Part model, mm, in its own coordinate system. A direction names the side the tool comes from. Round coordinates to 2 decimals unless told otherwise and drop trailing zeros. Write each loop counter-clockwise with the first axis right and the second up, starting at its lowest first coordinate (ties: lowest second). Pieces come first, ordered by that corner, then holes. Notation, with made-up numbers: M 88.25,63 L 128.25,63 A20 cw 128.25,79 Z; hole C 19,-16 d10. An arc over 180 degrees is marked long. Answer as a JSON object with one key per item and string values. Group by question number.
1. Band-saw the part on B-B, the plane x = 84. Write the cut outline in (y, z), plus the area to 3 significant figures.
2. Band-saw the part on A-A, the plane z = 8.25. Write the cut outline in (x, y).
3. Band-saw the part on C-C, the plane y = 62.5. Write the cut outline in (x, z), plus the area to 3 significant figures.
4. Drill centre lines: line 1 (Y direction, x = 192.5, z = 6.25); line 2 (X direction, y = 66, z = 11.5); line 3 (Z direction, x = 94, y = 80). Where is each one in solid material? Low to high. Write a range as from..to.
5. Two-plate mould, pull along Y, no slides. Class faces 4 (the face through (169, 4, 14.5)), 5 (the face through (181, 0.082, 9)), 6 (the face through (181, 89, 3)): +Y half, -Y half, draft (parallel to the pull), parting line (faces both ways), or undercut.
6. Which spindle directions (+Z, -Z, +X, -X, +Y, -Y) get a long thin tool onto all of the face, cutting with end or side? Do faces 1 (the face through (181, 176.492, 9)), 2 (the face through (367.772, 87, 9)), 3 (the face through (7.792, 87, 9)). Say none if no direction does.
7. Drop flat-ended pins along their axis: pin 1 (4 mm diameter, centred on y = 128, z = 6, fed in from +X); pin 2 (8 mm diameter, centred on x = 80, y = 72, fed in from +Z); pin 3 (6 mm diameter, centred on x = 138, z = 8, fed in from +Y). Give the stop position or say it passes through.
from build123d import *

# Parameters (mm, degrees)
SKETCH_5_W          = 383.47
SKETCH_5_H          = 192.04
EXTRUDE_2_DEPTH     = 3
EXTRUDE_START       = 3
SKETCH_6_W          = 367.88
SKETCH_6_H          = 176.41
EXTRUDE_3_DEPTH     = 11.5
CUT_EXTRUDE_START   = 14.5
SKETCH_7_W          = 352.07
SKETCH_7_H          = 160.62
CUT_EXTRUDE_1_DEPTH = 11.5


with BuildPart() as part:
    # 草图5 → 凸台-拉伸2 (new body)
    with BuildSketch(Plane.XY):
        with Locations((183.815306963, 88.27515573)):
            Rectangle(SKETCH_5_W, SKETCH_5_H)
    extrude(amount=EXTRUDE_2_DEPTH)

    # 草图6 → 凸台-拉伸3 (add)
    with BuildSketch(Plane.XY.offset(EXTRUDE_START)):
        with Locations((183.832314811, 88.286576554)):
            Rectangle(SKETCH_6_W, SKETCH_6_H)
    extrude(amount=EXTRUDE_3_DEPTH)

    # 草图7 → 切除-拉伸1 (cut)
    with BuildSketch(Plane.XY.offset(CUT_EXTRUDE_START)):
        with Locations((183.827427543, 88.282627)):
            Rectangle(SKETCH_7_W, SKETCH_7_H)
    extrude(amount=-CUT_EXTRUDE_1_DEPTH, mode=Mode.SUBTRACT)


solid = part.part
Worked answers:
{
 "1": {"outline": "M -7.74,0 L 184.3,0 L 184.3,3 L 176.49,3 L 176.49,14.5 L 168.59,14.5 L 168.59,3 L 7.97,3 L 7.97,14.5 L 0.08,14.5 L 0.08,3 L -7.74,3 Z", "area": "758 mm^2"},
 "2": {"outline": "M -0.11,0.08 L 367.77,0.08 L 367.77,176.49 L -0.11,176.49 Z; hole M 7.79,7.97 L 359.86,7.97 L 359.86,168.59 L 7.79,168.59 Z"},
 "3": {"outline": "M -7.92,0 L 375.55,0 L 375.55,3 L 367.77,3 L 367.77,14.5 L 359.86,14.5 L 359.86,3 L 7.79,3 L 7.79,14.5 L -0.11,14.5 L -0.11,3 L -7.92,3 Z", "area": "1,330 mm^2"},
 "4": {"line 1": "y = 0.08..7.97, 168.59..176.49", "line 2": "x = -0.11..7.79, 359.86..367.77", "line 3": "z = 0..3"},
 "5": {"face 4": "draft", "face 5": "-Y half", "face 6": "undercut"},
 "6": {"face 1": "+Z, +X, -X, +Y", "face 2": "+Z, +X, +Y, -Y", "face 3": "+Z"},
 "7": {"pin 1": "stops at x = 367.77", "pin 2": "stops at z = 3", "pin 3": "stops at y = 176.49"}
}
